Autodesk Inventor part; units mm, degrees
ref_plane "YZ Plane" through (0, 0, 0) normal (1, 0, 0) x (0, 1, 0)
ref_plane "XZ Plane" through (0, 0, 0) normal (0, 1, 0) x (-1, 0, 0)
ref_plane "XY Plane" through (0, 0, 0) normal (0, 0, 1) x (1, 0, 0)
sketch "Sketch1" plane through (0, 0, 0) normal (0, 0, 1) x (1, 0, 0)
  circle A0 centre (0, 0) radius 5
  circle A1 centre (0, 0) radius 7
  dimension "d0" = 10
  dimension "d1" = 14
extrude "Extrusion1" add sketch "Sketch1" along normal blind 10
sketch "Sketch2" plane through (0, 0, 10) normal (0, 0, 1) x (1, 0, 0)
  line L0 (-30, -27.5) -> (19.666, -27.5)
  line L1 (19.666, -27.5) -> (19.666, 27.5)
  line L2 (19.666, 27.5) -> (-30, 27.5)
  line L3 (-30, 27.5) -> (-30, -27.5)
  point P0 (0, 0)
  point P1 (-30, 0)
  dimension "d4" = 19.666
  dimension "d5" = 55
  dimension "d6" = 30
extrude "Extrusion2" add sketch "Sketch2" along normal blind 50
sketch "Sketch3" plane through (0, 0, 10) normal (0, 0, -1) x (-1, 0, 0)
  circle A0 centre (0, 0) radius 5
extrude "Extrusion3" cut sketch "Sketch3" against normal up to surface (50 mm away)
properties part number "02BombaJarron"
The model under review builds one solid part; all positions refer to its coordinate system, in mm. A direction names the side the tool comes from. Give positions to 0.01 mm unless a question says otherwise; leave off trailing zeros. Loops run counter-clockwise (first coordinate to the right, second up) from the corner with the lowest first, then second, coordinate; pieces in that order, holes last. Notation, with made-up numbers: (2, -19.5) -> (29, -19.5) arc R22 cw to (29, 16.5) -> close; hole circle Ø1 at (81, 13). An arc over 180 degrees is marked (long way). Put each result on its own line as item: value. Start each with the question number.
1. We need section B-B on x = 0. State the section outline as (y, z) points, then the cut area to 3 significant figures.
2. For faces 1 (the face through (6.466, 2.681, 4.93)), 2 (the face through (19.666, 0, 35)), list the 3-axis set-ups (+Z, -Z, +X, -X, +Y, -Y) from which the entire face can be reached by the end or side of a thin tool; tool diameter is ignored.
3. We need section D-D on y = -19. State the section outline as (x, z) points.
4. Wall thickness on probe 1 along X at (y, z) = (0, 47); probe 2 along Y at (x, z) = (0, 40.5); probe 3 along Z at (x, y) = (2.5, -7): over which ranges is each line inside the solid? List them lowest first.
5. We need section C-C on z = 49.5. State the section outline as (x, y) points, then the cut area to 3 significant figures.
6. We need section A-A on y = 0. State the section outline as (x, z) points.
Determined:
1. outline: (-27.5, 10) -> (-7, 10) -> (-7, 0) -> (-5, 0) -> (-5, 60) -> (-27.5, 60) -> close; (5, 0) -> (7, 0) -> (7, 10) -> (27.5, 10) -> (27.5, 60) -> (5, 60) -> close
1. area: 2,290 mm^2
2. face 1: -Z
2. face 2: +Z, -Z, +X, +Y, -Y
3. outline: (-30, 10) -> (19.67, 10) -> (19.67, 60) -> (-30, 60) -> close
4. probe 1: -30 to -5, 5 to 19.67
4. probe 2: -27.5 to -5, 5 to 27.5
4. probe 3: 10 to 60
5. outline: (-30, -27.5) -> (19.67, -27.5) -> (19.67, 27.5) -> (-30, 27.5) -> close; hole circle Ø10 at (0, 0)
5. area: 2,650 mm^2
6. outline: (-30, 10) -> (-7, 10) -> (-7, 0) -> (-5, 0) -> (-5, 60) -> (-30, 60) -> close; (5, 0) -> (7, 0) -> (7, 10) -> (19.67, 10) -> (19.67, 60) -> (5, 60) -> close
